from build123d import *

# Parameters (mm, degrees)
EXTRUDE_1_DEPTH = 8
FILLET_1_R      = 8
FILLET_2_R      = 20


with BuildPart() as part:
    # 草图1 → 凸台-拉伸1 (new body)
    with BuildSketch(Plane.XY):
        Polygon((0, 0), (0, 114), (-27, 114), (-27, 139), (-73, 139), (-73, 30), (-45, 0), align=None)
    extrude(amount=EXTRUDE_1_DEPTH)

    # 圆角1
    fillet_1_edges = [part.edges().sort_by_distance(p)[0] for p in [
        (-73, 139, 4),
    ]]
    fillet(fillet_1_edges, radius=FILLET_1_R)

    # 圆角2
    fillet_2_edges = [part.edges().sort_by_distance(p)[0] for p in [
        (-45, 0, 4),
        (-73, 30, 4),
    ]]
    fillet(fillet_2_edges, radius=FILLET_2_R)


solid = part.part
The listing builds one solid part. Answer for the finished solid, in the listing's coordinates (mm). A direction names the side the tool comes from. Give positions to 0.01 mm unless a question says otherwise; leave off trailing zeros. Write each loop counter-clockwise with the first axis right and the second up, starting at its lowest first coordinate (ties: lowest second). Pieces come first, ordered by that corner, then holes.
1) Section C-C (x = -4) is taken. Write down the section's boundary in (y, z), and give its area (3 significant figures).
2) A tool of negligible diameter and unlimited length cuts with its end or side. For faces 1 (the face through (-27, 126, 4)), 2 (the face through (-70.594, 136.719, 4.056)), from which of +Z, -Z, +X, -X, +Y, -Y can it reach the whole face along a straight path? Write none if from no direction.
3) Section A-A (z = 1.75) is taken. Write down the section's boundary in (x, y), and give its area (3 significant figures).
4) Given P1, Ø1, axis at y = 29.5, z = 3.5, coming from the +X side; P2, Ø1, axis at x = -65.5, z = 6.5, coming from the -Y side; P3, Ø4, axis at y = 131.5, z = 2.5, coming from the +X side, each flat-ended and moving along its own axis, determine where each tip first touches the part or whether it passes through.
5) Section B-B (y = 117) is taken. Write down the section's boundary in (x, z).
6) Find the intervals of material crossed by L1, parallel to Y at x = -21, z = 4.25; L2, parallel to X at y = 124, z = 4; L3, parallel to Y at x = -47.5, z = 4, in increasing order.
Response:
1. outline: (0, 0) - (114, 0) - (114, 8) - (0, 8) - close
1. area: 912 mm2
2. face 1: +Z, -Z, +X, +Y
2. face 2: +Z, -Z, -X, +Y
3. outline: (-73, 37.88) arc R20 ccw to (-67.62, 24.24) - (-50.93, 6.35) arc R20 ccw to (-36.31, 0) - (0, 0) - (0, 114) - (-27, 114) - (-27, 139) - (-65, 139) arc R8 ccw to (-73, 131) - close
3. area: 9,020 mm2
4. P1: stops at x = 0
4. P2: stops at y = 21.43
4. P3: stops at x = -27
5. outline: (-73, 0) - (-27, 0) - (-27, 8) - (-73, 8) - close
6. L1: y = 0 to 114
6. L2: x = -73 to -27
6. L3: y = 3.42 to 139
